Geometry: see drawing. Coordinates: mm, zero at the bounding-box minimum. Round coordinates to 2 decimals unless told otherwise and drop trailing zeros. Loops run counter-clockwise (first coordinate to the right, second up) from the corner with the lowest first, then second, coordinate; pieces in that order, holes last. Notation, with made-up numbers: (17, 63.5) -> (76, 63.5) arc R17 ccw to (76, 84.5) -> close; hole circle Ø7 at (24.25, 76.5). An arc over 180 degrees is marked (long way). Answer in a Markdown table with one row per item.
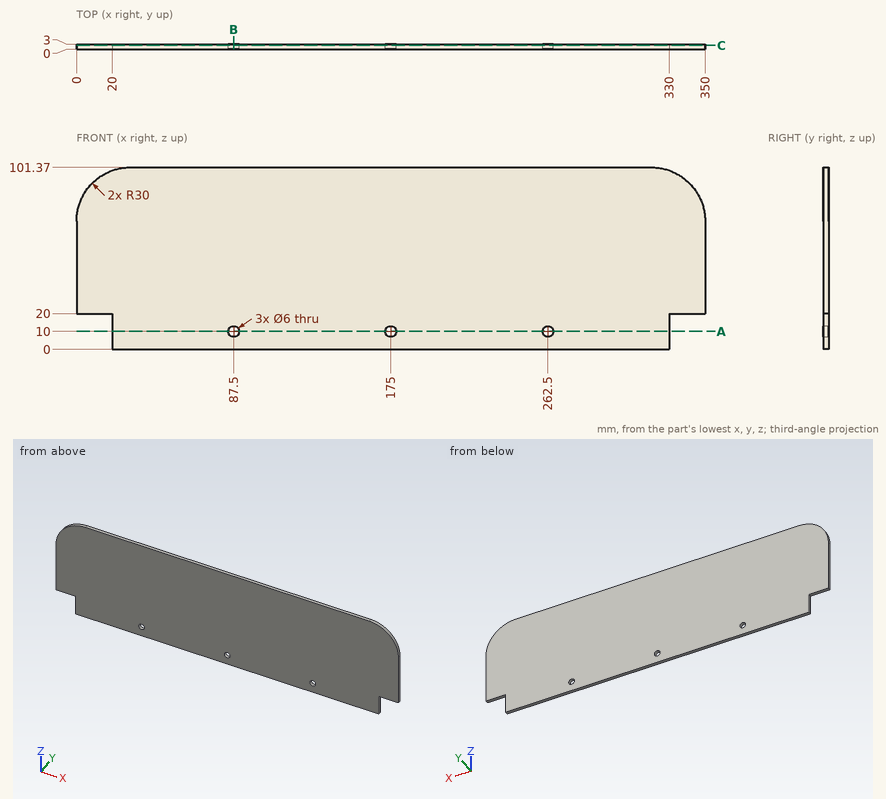
Item 1: Section query C-C, the plane y = 2.3. Output: boundary loops of the cut face in (x, z).
Ans:
| item | result |
|---|---|
| outline | (0, 20) -> (20, 20) -> (20, 0) -> (330, 0) -> (330, 20) -> (350, 20) -> (350, 71.37) arc R30 ccw to (320, 101.37) -> (30, 101.37) arc R30 ccw to (0, 71.37) -> close; hole circle Ø6 at (87.5, 10); hole circle Ø6 at (175, 10); hole circle Ø6 at (262.5, 10) |
Item 2: Section query B-B, the plane x = 87.5. Output: boundary loops of the cut face in (y, z), and give its area (3 significant figures).
Ans:
| item | result |
|---|---|
| outline | (0, 0) -> (3, 0) -> (3, 7) -> (0, 7) -> close; (0, 13) -> (3, 13) -> (3, 101.37) -> (0, 101.37) -> close |
| area | 286 mm2 |
Item 3: Section query A-A, the plane z = 10. Output: boundary loops of the cut face in (x, y), and give its area (3 significant figures).
Ans:
| item | result |
|---|---|
| outline | (20, 0) -> (84.5, 0) -> (84.5, 3) -> (20, 3) -> close; (90.5, 0) -> (172, 0) -> (172, 3) -> (90.5, 3) -> close; (178, 0) -> (259.5, 0) -> (259.5, 3) -> (178, 3) -> close; (265.5, 0) -> (330, 0) -> (330, 3) -> (265.5, 3) -> close |
| area | 876 mm2 |
Item 4: Ray query, L1, parallel to X at y = 1.8, z = 10; L2, parallel to X at y = 1.7, z = 18; L3, parallel to Z at x = 262.5, y = 1.75. Return the intervals inside material, ascending.
Ans:
| item | result |
|---|---|
| L1 | 20 to 84.5, 90.5 to 172, 178 to 259.5, 265.5 to 330 |
| L2 | 20 to 330 |
| L3 | 0 to 7, 13 to 101.37 |
Item 5: First-contact query: P1, Ø0.9, axis at y = 1, z = 7, coming from the -X side; P2, Ø1.5, axis at x = 10.5, y = 2, coming from the -Z side. Flat tips, straight axial feed; report the tip coordinate or a pass-through.
Ans:
| item | result |
|---|---|
| P1 | x = 20 |
| P2 | z = 20 |
